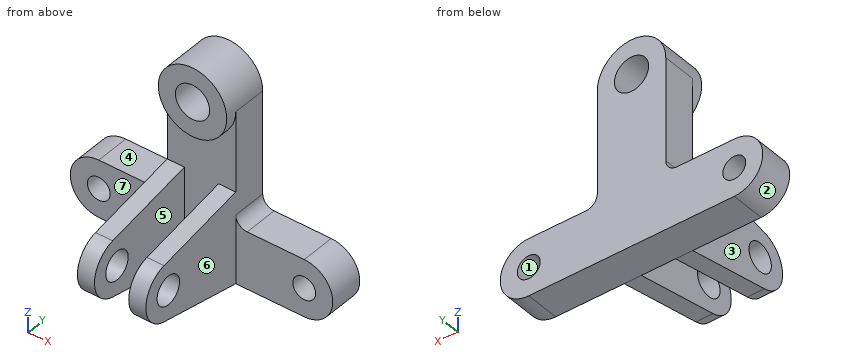
Solid Edge part; units mm, degrees
sketch "Sketch1" plane through (0, 0, 0) normal (0, -1, 0) x (1, 0, 0)
  line L0 (30, 150) -> (30, 80)
  line L1 (30, 80) -> (30, 60)
  line L2 (40, 50) -> (90, 50)
  line L3 (0, 0) -> (90, 0)
  line L4 (0, 0) -> (-90, 0)
  line L5 (-90, 50) -> (-40, 50)
  line L6 (-30, 60) -> (-30, 80)
  line L7 (-30, 80) -> (-30, 150)
  arc A0 (40, 50) -> (30, 60) centre (40, 60) cw
  arc A1 (90, 50) -> (90, 0) centre (90, 25) cw
  arc A2 (-90, 0) -> (-90, 50) centre (-90, 25) cw
  arc A3 (-30, 60) -> (-40, 50) centre (-40, 60) cw
  arc A4 (-30, 150) -> (30, 150) centre (0, 150) cw
  circle A5 centre (0, 150) radius 15
  circle A6 centre (-90, 25) radius 10
  arc A7 (90, 15) -> (90, 35) centre (90, 25) cw
  arc A8 (90, 35) -> (90, 15) centre (90, 25) cw
extrude "Protrusion1" add sketch "Sketch1" along normal mid plane 30
sketch "Sketch2" plane through (0, -15, 90) normal (0, -1, 0) x (1, 0, 0)
  circle A0 centre (0, 60) radius 30
  circle A1 centre (0, 60) radius 15
extrude "ExtrudedProtrusion_2" add sketch "Sketch2" along normal blind 10
sketch "Sketch3" plane through (30, 0, 0) normal (1, 0, 0) x (0, 1, 0)
  line L0 (-15, 80) -> (-94.7565, 64.5434)
  line L1 (-15, 40) -> (-15, 80)
  line L2 (-15, 0) -> (-15, 40)
  line L3 (-15, 0) -> (-94.7565, 15.4566)
  arc A0 (-94.7565, 15.4567) -> (-94.7565, 64.5433) centre (-90, 40) cw
  circle A1 centre (-90, 40) radius 12.5
extrude "Protrusion2" add sketch "Sketch3" against normal up to vertex (60 mm away)
sketch "Sketch4" plane through (0, -15, 115) normal (0, -1, 0) x (1, 0, 0)
  line L0 (-15, -35) -> (-15, -115)
  line L1 (-15, -115) -> (15, -115)
  line L2 (15, -115) -> (15, -35)
  line L3 (-15, -35) -> (15, -35)
extrude "ExtrudedCutout_1" cut sketch "Sketch4" along normal blind 222.03
Geometry check sheet. Reference: the model listing, model coordinates, mm. Face numbers are marked on the shaded views. A direction names the side the tool comes from. Coordinates: 2 decimals unless noted, no trailing zeros. Order: outer loops, then holes, each group sorted by start corner. A loop starts at its lowest first (then second) coordinate and runs counter-clockwise, first axis right, second up. Notation, with made-up numbers: M 87.5,-16 L 131.5,-16 A26 cw 131.5,19 Z; hole C -32,66 d11. An arc over 180 degrees is marked long. Use CSV: the item, a comma, the result in double quotes.
Item 1: Cross-section at C-C on y = -90. Record the cut outline in (x, z), then the cut area to 3 significant figures.
Returned:
outline,"M -30,14.53 L -15,14.53 L -15,27.5 L -30,27.5 Z; M -30,52.5 L -15,52.5 L -15,65.47 L -30,65.47 Z; M 15,14.53 L 30,14.53 L 30,27.5 L 15,27.5 Z; M 15,52.5 L 30,52.5 L 30,65.47 L 15,65.47 Z"
area,"778 mm2"
Item 2: Cross-section at A-A on x = 0. Record the cut outline in (y, z), then the cut area to 3 significant figures.
Returned:
outline,"M -25,120 L -15,120 L -15,0 L 15,0 L 15,135 L -25,135 Z; M -25,165 L 15,165 L 15,180 L -25,180 Z"
area,"4,800 mm2"
Item 3: Mould release check, pull along Z, two halves, no side actions. Record for the marked faces 1, 2 and 3: pulls with the +Z half, pulls with the -Z half, needs draft (parallel to the pull), parting line crosses it, or undercut.
Returned:
face 1,"undercut"
face 2,"parting line crosses it"
face 3,"needs draft"
Item 4: Thickness scan on line 1 along Z through (x, y) = (90, 0); line 2 along X through (y, z) = (-48.5, 10); line 3 along Z through (x, y) = (-89, 6.5). Record the ranges inside material, lowest first.
Returned:
line 1,"z = 0 to 15, 35 to 50"
line 2,"x = -30 to -15, 15 to 30"
line 3,"z = 0 to 15.05, 34.95 to 50"
Item 5: Gauge pin test, flat ends, axial feed: pin 1 Ø3 at (x, y) = (31, -85.5) entering from -Z; pin 2 Ø20 at (y, z) = (-90, 40) entering from -X; pin 3 Ø18 at (x, z) = (-11, 68.5) entering from -Y; pin 4 Ø1.5 at (y, z) = (-8, 90) entering from -X. Record the tip position at first contact, or that the pin passes through.
Returned:
pin 1,"stops at z = 13.45"
pin 2,"passes through"
pin 3,"stops at y = -104.4"
pin 4,"stops at x = -30"
Item 6: Cross-section at B-B on z = 40. Record the cut outline in (x, y), then the cut area to 3 significant figures.
Returned:
outline,"M -110,-15 L -30,-15 L -30,-77.5 L -15,-77.5 L -15,-15 L 15,-15 L 15,-77.5 L 30,-77.5 L 30,-15 L 110,-15 L 110,15 L -110,15 Z; M -30,-115 L -15,-115 L -15,-102.5 L -30,-102.5 Z; M 15,-115 L 30,-115 L 30,-102.5 L 15,-102.5 Z"
area,"8,850 mm2"
Item 7: Tool access check on the marked faces 4, 5, 6 and 7. Record the directions out of +Z, -Z, +X, -X, +Y, -Y that give a thin tool (end or side, any length) a straight path to the whole face; none if there is none.
Returned:
face 4,"+Z, -X, +Y, -Y"
face 5,"-Z, -Y"
face 6,"+Z, +X, -Y"
face 7,"+Z, -Z, -X, -Y"
Item 8: Cross-section at D-D on y = -64. Record the cut outline in (x, z), then the cut area to 3 significant figures.
Returned:
outline,"M -30,9.5 L -15,9.5 L -15,70.5 L -30,70.5 Z; M 15,9.5 L 30,9.5 L 30,70.5 L 15,70.5 Z"
area,"1,830 mm2"
